Design review of the part shown in the three views and the two pictorial views. Dimensions are in mm from the part's minimum x, y and z. A direction names the side the tool comes from. Round coordinates to 2 decimals unless told otherwise and drop trailing zeros. Order: outer loops, then holes, each group sorted by start corner. A loop starts at its lowest first (then second) coordinate and runs counter-clockwise, first axis right, second up.
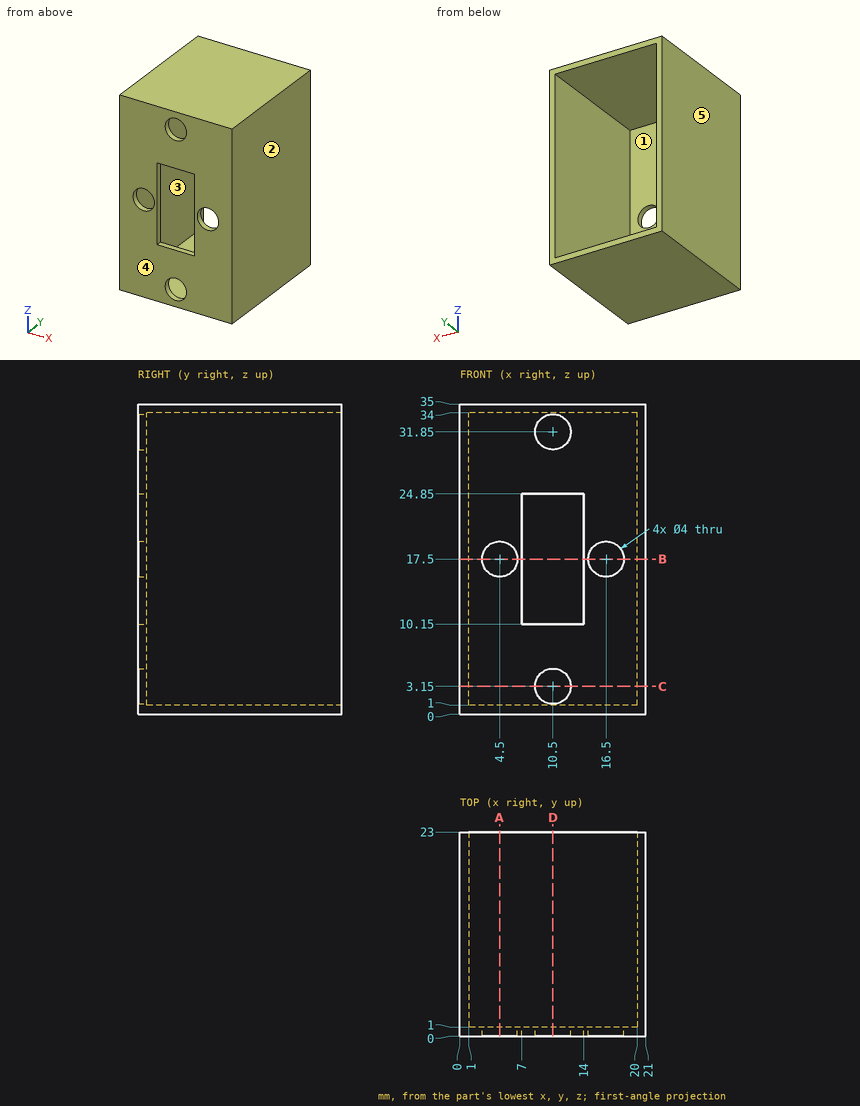
(1) Consider section B-B (z = 17.5). Write out the cut boundary in (x, y), and give its area (3 significant figures).
Data:
outline: (0, 0) - (2.5, 0) - (2.5, 1) - (1, 1) - (1, 23) - (0, 23) - close; (6.5, 0) - (7, 0) - (7, 1) - (6.5, 1) - close; (14, 0) - (14.5, 0) - (14.5, 1) - (14, 1) - close; (18.5, 0) - (21, 0) - (21, 23) - (20, 23) - (20, 1) - (18.5, 1) - close
area: 50.0 mm2
(2) Consider section D-D (x = 10.5). Write out the cut boundary in (y, z), and give its area (3 significant figures).
Data:
outline: (0, 0) - (23, 0) - (23, 1) - (1, 1) - (1, 1.15) - (0, 1.15) - close; (0, 5.15) - (1, 5.15) - (1, 10.15) - (0, 10.15) - close; (0, 24.85) - (1, 24.85) - (1, 29.85) - (0, 29.85) - close; (0, 33.85) - (1, 33.85) - (1, 34) - (23, 34) - (23, 35) - (0, 35) - close
area: 56.3 mm2
(3) For the marked faces 1 and 2, list the 3-axis set-ups (+Z, -Z, +X, -X, +Y, -Y) from which the entire face can be reached by the end or side of a thin tool; tool diameter is ignored.
Data:
face 1: +Y
face 2: +Z, -Z, +X, +Y, -Y
(4) Insertion check: pin 1 (4.5 mm diameter, centred on x = 16.5, z = 17.5, fed in from +Y); pin 2 (9.5 mm diameter, centred on x = 10, y = 11.5, fed in from -Z). Each pin has a flat end and moves straight along its axis. Give the tip position at first contact, or say it passes through.
Data:
pin 1: stops at y = 1
pin 2: stops at z = 0
(5) Consider section A-A (x = 4.5). Write out the cut boundary in (y, z), and give its area (3 significant figures).
Data:
outline: (0, 0) - (23, 0) - (23, 1) - (1, 1) - (1, 15.5) - (0, 15.5) - close; (0, 19.5) - (1, 19.5) - (1, 34) - (23, 34) - (23, 35) - (0, 35) - close
area: 75.0 mm2
(6) To check wall thickness, follow probe 1 along X at (y, z) = (18, 14); probe 2 along Z at (x, y) = (16.5, 0.35); probe 3 along Z at (x, y) = (6.75, 3.5). State the ranges of each line that lie inside material, in increasing order.
Data:
probe 1: x = 0 to 1, 20 to 21
probe 2: z = 0 to 15.5, 19.5 to 35
probe 3: z = 0 to 1, 34 to 35
(7) Consider section C-C (z = 3.15). Write out the cut boundary in (x, y), and give its area (3 significant figures).
Data:
outline: (0, 0) - (8.5, 0) - (8.5, 1) - (1, 1) - (1, 23) - (0, 23) - close; (12.5, 0) - (21, 0) - (21, 23) - (20, 23) - (20, 1) - (12.5, 1) - close
area: 61.0 mm2
(8) Draft analysis for pull direction X (two halves, no side actions). For the marked faces 3, 4 and 5, state which applies: pulls with the +X half, pulls with the -X half, needs draft (parallel to the pull), parting line crosses it, or undercut.
Data:
face 3: undercut
face 4: needs draft
face 5: pulls with the -X half
